from build123d import *

# Parameters (mm, degrees)
F1_DEPTH = 4.5
F2_W     = 0.5
F2_H     = 4.5
F3_DEPTH = 6
F4_W     = 0.5
F4_H     = 4.5
F5_DEPTH = 9
F6_W     = 0.6
F6_H     = 4.5
F7_DEPTH = 25


with BuildPart() as f1:
    # F0 (on Top) → F1 (new body)
    with BuildSketch(Plane.XY):
        Polygon((-0.469149, 31.306926), (-0.969149, 31.306926), (-0.969149, 8.820471), (-2.198889, 5.306926), (-2.198889, -1.893074), (-0.969149, -5.406618), (-0.969149, -26.693074), (-0.469149, -26.693074), (-0.469149, -5.406618), (0.760592, -1.893074), (0.760592, 5.306926), (-0.469149, 8.820471), align=None)
        Polygon((-1.669149, -1.893074), (-1.669149, 5.306926), (-0.969149, 7.306926), (-0.719149, 8.021212), (-0.469149, 7.306926), (0.230851, 5.306926), (0.230851, -1.893074), (-0.469149, -3.893074), (-0.719149, -4.607359), (-0.969149, -3.893074), align=None, mode=Mode.SUBTRACT)
    extrude(amount=F1_DEPTH)

    # F2 (on face) → F3 (join)
    with BuildSketch(Plane.XY.offset(4.5)):
        with Locations((-0.719149, 29.056926)):
            Rectangle(F2_W, F2_H)
    extrude(amount=F3_DEPTH)

    # F4 (on face) → F5 (join)
    with BuildSketch(Plane.XY.offset(4.5)):
        with Locations((-0.219149, -24.443074)):
            Rectangle(F4_W, F4_H)
        with Locations((-1.219149, -24.443074)):
            Rectangle(F4_W, F4_H)
    extrude(amount=-F5_DEPTH)

    # F6 (on face) → F7 (cut)
    with BuildSketch(Plane(origin=(0, 0, 0), x_dir=(1, 0, 0), z_dir=(0, 0, -1))):
        with Locations((-0.719149, 24.443074)):
            Rectangle(F6_W, F6_H)
    extrude(amount=F7_DEPTH, mode=Mode.SUBTRACT)


solid = f1.part
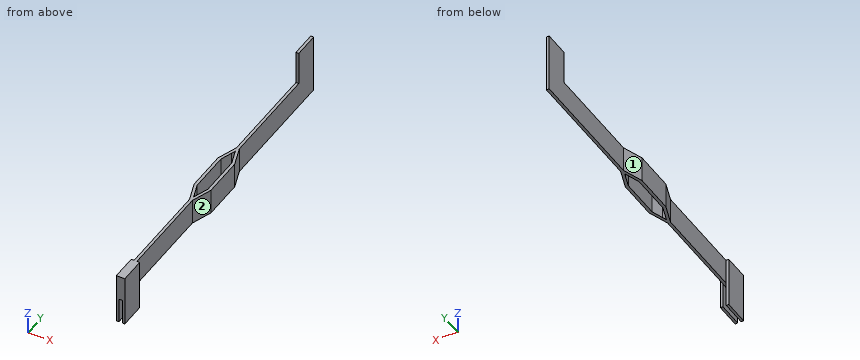
Verification items for the finished model (mm, model axes). Face numbers are marked on the shaded views. Give positions to 0.01 mm unless a question says otherwise; leave off trailing zeros. Write each loop counter-clockwise with the first axis right and the second up, starting at its lowest first coordinate (ties: lowest second). Pieces come first, ordered by that corner, then holes. Notation, with made-up numbers: M 8,7.25 L 26,7.25 A12 ccw 26,21.25 Z; hole C 59.25,16.5 d1. An arc over 180 degrees is marked long. Write item = value, one per line.
(1) Material ranges on line 1 (X direction, y = 13, z = 0.5); line 2 (Z direction, x = -0.8, y = -18); line 3 (Y direction, x = -1.25, z = -2.75), recorded low to high.
Found:
line_1 = -0.97 to -0.47
line_2 = 0 to 4.5
line_3 = -26.69 to -22.19
(2) Sectioned sample at C-C (y = -12). Record the cut outline in (x, z), then the cut area to 3 significant figures.
Found:
outline = M -0.97,0 L -0.47,0 L -0.47,4.5 L -0.97,4.5 Z
area = 2.25 mm2
(3) Draft check along Y on the marked faces 1 and 2. Enter one of: released by +Y, released by -Y, zero draft, split by the parting line, or undercut.
Found:
face_1 = released by +Y
face_2 = undercut
(4) Go/stop test with flat-tipped pins: pin 1 Ø1.3 at (y, z) = (-25, -2.5) entering from +X; pin 2 Ø1.5 at (x, y) = (-1, 1) entering from -Z; pin 3 Ø2 at (y, z) = (-25, -1.5) entering from -X. Record where each tip stops, or that it passes through.
Found:
pin_1 = 0.03
pin_2 = 0
pin_3 = -1.47
(5) Sectioned sample at D-D (z = 9). Record the cut outline in (x, y), then the cut area to 3 significant figures.
Found:
outline = M -0.97,26.81 L -0.47,26.81 L -0.47,31.31 L -0.97,31.31 Z
area = 2.25 mm2
(6) Sectioned sample at B-B (z = -1.75). Record the cut outline in (x, y), then the cut area to 3 significant figures.
Found:
outline = M -1.47,-26.69 L -1.02,-26.69 L -1.02,-22.19 L -1.47,-22.19 Z; M -0.42,-26.69 L 0.03,-26.69 L 0.03,-22.19 L -0.42,-22.19 Z
area = 4.05 mm2
(7) Sectioned sample at A-A (z = 3). Record the cut outline in (x, y), then the cut area to 3 significant figures.
Found:
outline = M -2.2,-1.89 L -0.97,-5.41 L -0.97,-22.19 L -1.47,-22.19 L -1.47,-26.69 L 0.03,-26.69 L 0.03,-22.19 L -0.47,-22.19 L -0.47,-5.41 L 0.76,-1.89 L 0.76,5.31 L -0.47,8.82 L -0.47,31.31 L -0.97,31.31 L -0.97,8.82 L -2.2,5.31 Z; hole M -1.67,-1.89 L -0.97,-3.89 L -0.72,-4.61 L -0.47,-3.89 L 0.23,-1.89 L 0.23,5.31 L -0.47,7.31 L -0.72,8.02 L -0.97,7.31 L -1.67,5.31 Z
area = 41.0 mm2
